from build123d import *

# Parameters (mm, degrees)
SKETCH_1_W               = 455
SKETCH_1_H               = 50
EXTRUDE_1_DEPTH          = 20
SKETCH_2_R               = 15
CUT_EXTRUDE_1_DEPTH      = 230.741702788
CUT_EXTRUDE_2_REACH      = 458.125
CUT_EXTRUDE_2_END_RADIUS = 15
SKETCH_3_R               = 6
CHAMFER_1_SIZE           = 0.5
CHAMFER_2_SIZE           = 0.5
FILLET_1_R               = 10


with BuildPart() as part:
    # 草图1 → 凸台-拉伸1 (new body)
    with BuildSketch(Plane(origin=(0, 0, 0), x_dir=(1, 0, 0), z_dir=(0, 1, 0))):
        Rectangle(SKETCH_1_W, SKETCH_1_H)
    extrude(amount=EXTRUDE_1_DEPTH)

    # 草图2 → 切除-拉伸1 (cut, through all)
    with BuildSketch(Plane(origin=(0, 20, 0), x_dir=(1, 0, 0), z_dir=(0, 1, 0))):
        with Locations(Location((-192.5, 0, 0), (0, 0, 270))):
            Circle(SKETCH_2_R)
        with Locations(Location((-122.5, 0, 0), (0, 0, 270))):
            Circle(SKETCH_2_R)
        with Locations(Location((-52.5, 0, 0), (0, 0, 270))):
            Circle(SKETCH_2_R)
        with BuildLine():
            Line((31.5, 15), (191.5, 15))
            ThreePointArc((191.5, 15), (206.5, 0), (191.5, -15))
            Line((191.5, -15), (31.5, -15))
            ThreePointArc((31.5, -15), (16.5, 0), (31.5, 15))
        make_face()
    extrude(amount=-CUT_EXTRUDE_1_DEPTH, mode=Mode.SUBTRACT)

    # 切除-拉伸2: up to this cylinder (the profile starts outside it)
    cut_extrude_2_end = Plane(origin=(191.5, 10, 0), z_dir=(0, 1, 0)) * Cylinder(CUT_EXTRUDE_2_END_RADIUS, 947.25, mode=Mode.PRIVATE)
    # 草图3 → 切除-拉伸2 (cut, up to the surface)
    with BuildSketch(Plane(origin=(227.5, 0, 0), x_dir=(0, 0, -1), z_dir=(1, 0, 0)), mode=Mode.PRIVATE) as cut_extrude_2_sk1:
        with Locations((0, 10)):
            Circle(SKETCH_3_R)
    cut_extrude_2_tool1 = extrude(cut_extrude_2_sk1.sketch, amount=-CUT_EXTRUDE_2_REACH, mode=Mode.PRIVATE) - cut_extrude_2_end
    add(cut_extrude_2_tool1.solids().sort_by_distance((227.5, 10, 0))[0], mode=Mode.SUBTRACT)

    # 倒角1
    chamfer_1_edges = [part.edges().sort_by_distance(p)[0] for p in [
        (-192.5, 0, -15),
        (-192.5, 20, -15),
        (-122.5, 0, -15),
        (-122.5, 20, -15),
        (-52.5, 0, -15),
        (-52.5, 20, -15),
        (16.5, 0, 0),
        (111.5, 0, -15),
        (206.5, 0, 0),
        (111.5, 0, 15),
        (16.5, 20, 0),
        (111.5, 20, 15),
        (206.5, 20, 0),
        (111.5, 20, -15),
    ]]
    chamfer(chamfer_1_edges, length=CHAMFER_1_SIZE)

    # 倒角2
    chamfer_2_edges = [part.edges().sort_by_distance(p)[0] for p in [
        (0, 20, -25),
        (-227.5, 20, 0),
        (0, 0, -25),
        (227.5, 0, 0),
        (0, 0, 25),
        (-227.5, 0, 0),
        (0, 20, 25),
    ]]
    chamfer(chamfer_2_edges, length=CHAMFER_2_SIZE)

    # 圆角1
    # the kernel refuses this fillet: 10 mm, written as the material it takes off along each edge
    with BuildSketch(Plane(origin=(227.5, -24.5, 25), x_dir=(0, 0, -1), z_dir=(0, 1, 0)), Plane(origin=(227.5, -24.5, -25), x_dir=(-1, 0, 0), z_dir=(0, 1, 0))) as fillet_1_piece_1:
        with BuildLine():
            CenterArc((FILLET_1_R, FILLET_1_R), FILLET_1_R, 180, 90)
            Line((0, FILLET_1_R), (0, 0))
            Line((0, 0), (FILLET_1_R, 0))
        make_face()
    extrude(amount=69, mode=Mode.SUBTRACT)
    with BuildSketch(Plane(origin=(-227.5, -24.5, -25), x_dir=(1, 0, 0), z_dir=(0, 1, 0)), Plane(origin=(-227.5, -24.5, 25), x_dir=(0, 0, -1), z_dir=(0, 1, 0))) as fillet_1_piece_2:
        with BuildLine():
            CenterArc((FILLET_1_R, -FILLET_1_R), FILLET_1_R, 90, 90)
            Line((0, -FILLET_1_R), (0, 0))
            Line((0, 0), (FILLET_1_R, 0))
        make_face()
    extrude(amount=69, mode=Mode.SUBTRACT)


solid = part.part
Here's how the part is built. I have some questions about the finished solid (model axes, mm). A direction names the side the tool comes from. Coordinates: 2 decimals unless noted, no trailing zeros. Write each loop counter-clockwise with the first axis right and the second up, starting at its lowest first coordinate (ties: lowest second). Pieces come first, ordered by that corner, then holes.
1) Which directions (+Z, -Z, +X, -X, +Y, -Y) give clear straight access to the entire face, cutting with the end or side of a thin tool? Please do faces 1 (the face through (216.529, 4.143, 1.301)), 2 (the face through (113, 10, 15)), 3 (the face through (16.368, 19.635, 0.333)), 4 (the face through (-224.49, 9.86, -22.15)).
Filled in:
face 1: +X
face 2: +Y, -Y
face 3: +Y
face 4: -Z, -X, +Y, -Y
2) If we section it at B-B (y = 10): List the corners of the cut face in (x, z) for me, plus the area to 3 significant figures.
Filled in:
outline: (-227.5, -15) arc R10 ccw to (-217.5, -25) - (217.5, -25) arc R10 ccw to (227.5, -15) - (227.5, -6) - (205.25, -6) arc R15 cw to (191.5, -15) - (31.5, -15) arc R15 cw to (31.5, 15) - (191.5, 15) arc R15 cw to (205.25, 6) - (227.5, 6) - (227.5, 15) arc R10 ccw to (217.5, 25) - (-217.5, 25) arc R10 ccw to (-227.5, 15) - close; hole circle Ø30 at (-192.5, 0); hole circle Ø30 at (-122.5, 0); hole circle Ø30 at (-52.5, 0)
area: 14,800 mm2
3) If I drill on line 1 (X direction, y = 8.5, z = 1.5); line 2 (X direction, y = 6.5, z = 0); line 3 (X direction, y = 1.25, z = -1.5), over which ranges is the centre line in solid material (lowest first)?
Filled in:
line 1: x = -227.5 to -207.42, -177.58 to -137.42, -107.58 to -67.42, -37.58 to 16.58
line 2: x = -227.5 to -207.5, -177.5 to -137.5, -107.5 to -67.5, -37.5 to 16.5
line 3: x = -227.5 to -207.42, -177.58 to -137.42, -107.58 to -67.42, -37.58 to 16.58, 206.42 to 227.5
4) If we section it at A-A (x = -122.5): List the corners of the cut face in (y, z) for me, plus the area to 3 significant figures.
Filled in:
outline: (0, -24.5) - (0.5, -25) - (19.5, -25) - (20, -24.5) - (20, -15.5) - (19.5, -15) - (0.5, -15) - (0, -15.5) - close; (0, 15.5) - (0.5, 15) - (19.5, 15) - (20, 15.5) - (20, 24.5) - (19.5, 25) - (0.5, 25) - (0, 24.5) - close
area: 399 mm2
5) Thinking about a two-plate mould opening in Z: for faces 5 (the face through (224.65, 9.86, -21.99)), 6 (the face through (16.368, 0.365, -0.333)), 7 (the face through (-224.65, 9.86, 21.99)), which applies, +Z half, -Z half, draft (parallel to the pull), parting line (faces both ways), or undercut?
Filled in:
face 5: -Z half
face 6: undercut
face 7: +Z half
6) I'm going to push flat-ended pins straight in: pin 1 (18 mm diameter, centred on x = -52.5, z = 0, fed in from +Y); pin 2 (7 mm diameter, centred on y = 10, z = 0, fed in from +X); pin 3 (1 mm diameter, centred on y = 13, z = 18, fed in from +X). Where does each tip first touch, or does it pass through?
Filled in:
pin 1: passes through
pin 2: stops at x = 16.91
pin 3: stops at x = 227.18
7) If we section it at C-C (z = 0): Count the separate pieces of the cut face and the enclosed holes in it, plus the area to 3 significant figures.
Filled in:
separate pieces: 6
enclosed holes: 0
area: 3,250 mm2
